CAD build for the part. Positions are in the model's coordinates, mm. A direction names the side the tool comes from. Give positions to 0.01 mm unless a question says otherwise; leave off trailing zeros. Write each loop counter-clockwise with the first axis right and the second up, starting at its lowest first coordinate (ties: lowest second). Pieces come first, ordered by that corner, then holes. Notation, with made-up numbers: (-8.75, 60.25) - (48.25, 60.25) arc R27 cw to (48.25, 76.25) - close; hole circle Ø2 at (61, 51). An arc over 180 degrees is marked (long way). Answer as a JSON object with one key per item and string values.
from build123d import *

# Parameters (mm, degrees)
BOSS_EXTRUDE1_DEPTH = 8
SKETCH10_W          = 20
SKETCH10_H          = 4.457955928
CUT_EXTRUDE1_DEPTH  = 8
SKETCH11_R          = 1.6
CUT_EXTRUDE2_DEPTH  = 17
CIRPATTERN1_START   = 27.11938858
CIRPATTERN1_DEPTH   = 8
FILLET1_R           = 4
SKETCH13_R          = 1.6
CUT_EXTRUDE3_DEPTH  = 4


# Read off the part's stored shape, not the designer's step: CirPattern1
with BuildPart() as part:
    # Sketch9 → Boss-Extrude1 (new body)
    with BuildSketch(Plane.XY.offset(35.11938858)):
        with BuildLine():
            Line((9.545521872, 41.744275524), (-57.430180647, 41.351233323))
            Line((-57.430180647, 41.351233323), (-12.111028973, 4.62462141))
            Line((-12.111028973, 4.62462141), (-5.395050947, -0.818002943))
            ThreePointArc((-5.395050947, -0.818002943), (4.336911047, 15.452862836), (9.11951655, 33.798948033))
            Line((9.11951655, 33.798948033), (11.42846507, 34.572240818))
            Line((11.42846507, 34.572240818), (11.499640251, 35.338944212))
            Line((11.499640251, 35.338944212), (9.372495407, 36.524051722))
            ThreePointArc((9.372495407, 36.524051722), (9.443412954, 37.633480095), (9.495906894, 38.743932705))
            Line((9.495906894, 38.743932705), (16.9130003, 38.787459396))
            Line((16.9130003, 38.787459396), (16.895395314, 41.78740774))
            Line((16.895395314, 41.78740774), (9.545521872, 41.744275524))
        make_face()
    extrude(amount=-BOSS_EXTRUDE1_DEPTH)

    # Sketch10 → Cut-Extrude1 (cut)
    with BuildSketch(Plane.XY.offset(35.11938858)):
        with Locations((-23.032343606, 36.517264559)):
            Rectangle(SKETCH10_W, SKETCH10_H)
    extrude(amount=-CUT_EXTRUDE1_DEPTH, mode=Mode.SUBTRACT)

    # Sketch11 → Cut-Extrude2 (cut)
    with BuildSketch(Plane(origin=(0.747199109, 41.914596091, 0), x_dir=(0.9998411421690517, -0.01782387236506677, 0), z_dir=(0.01782387236506677, 0.9998411421690517, 0))):
        with Locations(Location((-23.320690328, -31.11938858, 0), (0, 0, 180))):
            Circle(SKETCH11_R)
    extrude(amount=-CUT_EXTRUDE2_DEPTH, mode=Mode.SUBTRACT)

    # CirPattern1 outline → CirPattern1 (add)
    with BuildSketch(Plane.XY.offset(CIRPATTERN1_START)):
        with BuildLine():
            Line((-1.898240417, 0.075678285), (-1.442349939, 0.696213436))
            Line((-1.442349939, 0.696213436), (-2.655293453, 2.807609427))
            ThreePointArc((-2.655293453, 2.807609427), (-3.454215375, 1.696544027), (-4.275670815, 0.602033397))
            Line((-4.275670815, 0.602033397), (-1.898240417, 0.075678285))
        make_face()
        with BuildLine():
            ThreePointArc((9.087032741, 33.518000709), (8.913106654, 32.160616358), (8.711484025, 30.807068844))
            Line((8.711484025, 30.807068844), (11.052940174, 31.475505904))
            Line((11.052940174, 31.475505904), (11.158600181, 32.238222079))
            Line((11.158600181, 32.238222079), (9.087032741, 33.518000709))
        make_face()
        with BuildLine():
            ThreePointArc((8.666370259, 30.527871164), (8.431440362, 29.179705557), (8.169015006, 27.836621236))
            Line((8.169015006, 27.836621236), (10.538219647, 28.398843937))
            Line((10.538219647, 28.398843937), (10.678149721, 29.156022631))
            Line((10.678149721, 29.156022631), (8.666370259, 30.527871164))
        make_face()
        with BuildLine():
            ThreePointArc((8.11136298, 27.559740684), (7.81590678, 26.223534041), (7.493212091, 24.893642806))
            Line((7.493212091, 24.893642806), (9.885349689, 25.348508399))
            Line((9.885349689, 25.348508399), (10.059265414, 26.098610606))
            Line((10.059265414, 26.098610606), (8.11136298, 27.559740684))
        make_face()
        with BuildLine():
            ThreePointArc((7.423138984, 24.619642155), (7.067757013, 23.298110387), (6.685448884, 21.984115313))
            Line((6.685448884, 21.984115313), (9.095657291, 22.330699261))
            Line((9.095657291, 22.330699261), (9.303205175, 23.072200358))
            Line((9.303205175, 23.072200358), (7.423138984, 24.619642155))
        make_face()
        with BuildLine():
            ThreePointArc((6.603097126, 21.713551487), (6.188511716, 20.409380678), (5.74736721, 19.113952531))
            Line((5.74736721, 19.113952531), (8.170747547, 19.351550382))
            Line((8.170747547, 19.351550382), (8.411505736, 20.082943228))
            Line((8.411505736, 20.082943228), (6.603097126, 21.713551487))
        make_face()
        with BuildLine():
            ThreePointArc((5.652904183, 18.847375463), (5.179958002, 17.563216411), (4.680873768, 16.288988219))
            Line((4.680873768, 16.288988219), (7.112500384, 16.417117043))
            Line((7.112500384, 16.417117043), (7.385979526, 17.136915042))
            Line((7.385979526, 17.136915042), (5.652904183, 18.847375463))
        make_face()
        with BuildLine():
            ThreePointArc((4.574491474, 16.026939742), (4.04414581, 14.76540257), (3.488136265, 13.514964269))
            Line((3.488136265, 13.514964269), (5.923066749, 13.533363638))
            Line((5.923066749, 13.533363638), (6.228710981, 14.240103762))
            Line((6.228710981, 14.240103762), (4.574491474, 16.026939742))
        make_face()
        with BuildLine():
            ThreePointArc((3.370050932, 13.257977012), (2.783383741, 12.021625861), (2.171579003, 10.797519035))
            Line((2.171579003, 10.797519035), (4.604864227, 10.70615155))
            Line((4.604864227, 10.70615155), (4.942052312, 11.398397312))
            Line((4.942052312, 11.398397312), (3.370050932, 13.257977012))
        make_face()
        with BuildLine():
            ThreePointArc((2.042030645, 10.546115336), (1.400234361, 9.337463157), (0.733877956, 8.142175869))
            Line((0.733877956, 8.142175869), (3.160572137, 7.94122724))
            Line((3.160572137, 7.94122724), (3.528618722, 8.617571614))
            Line((3.528618722, 8.617571614), (2.042030645, 10.546115336))
        make_face()
        with BuildLine():
            ThreePointArc((0.593129889, 7.896866722), (-0.102491005, 6.718370166), (-0.82204467, 5.554331901))
            Line((-0.82204467, 5.554331901), (1.593126081, 5.244210567))
            Line((1.593126081, 5.244210567), (1.991283091, 5.903278845))
            Line((1.991283091, 5.903278845), (0.593129889, 7.896866722))
        make_face()
        with BuildLine():
            ThreePointArc((-0.973706371, 5.315615908), (-1.721737986, 4.169670332), (-2.493026381, 3.039247062))
            Line((-2.493026381, 3.039247062), (-0.094288024, 2.620583361))
            Line((-0.094288024, 2.620583361), (0.333170136, 3.261035952))
            Line((0.333170136, 3.261035952), (-0.973706371, 5.315615908))
        make_face()
    extrude(amount=CIRPATTERN1_DEPTH)

    # Fillet1
    fillet1_edges = [part.edges().sort_by_distance(p)[0] for p in [
        (-57.430180647, 41.351233323, 31.11938858),
    ]]
    fillet(fillet1_edges, radius=FILLET1_R)

    # Sketch13 → Cut-Extrude3 (cut)
    with BuildSketch(Plane(origin=(-0.244636188, 41.68682267, 0), x_dir=(0.9999827812112165, 0.005868328644527354, 0), z_dir=(-0.005868328644527354, 0.9999827812112165, 0))):
        with Locations(Location((12.140326638, -31.11938858, 0), (0, 0, 180))):
            Circle(SKETCH13_R)
    extrude(amount=-CUT_EXTRUDE3_DEPTH, mode=Mode.SUBTRACT)


solid = part.part
(1) Flat gauge pins, fed straight in: P1, Ø4, axis at x = -24.5, z = 30.5, coming from the +Y side; P2, Ø1.3, axis at y = 36.5, z = 31, coming from the +X side; P3, Ø4, axis at x = -23.5, z = 30.5, coming from the -Y side. Where does each tip first touch, or does it go through?
Answer key:
{"P1": "stops at y = 41.55", "P2": "stops at x = 10.58", "P3": "stops at y = 12.23"}
(2) Probe L1, parallel to Y at x = -20.5, z = 31; L2, parallel to Y at x = 11, z = 33.5; L3, parallel to Y at x = 9, z = 30.5. List the from-to ranges inside material, lowest first. Write a range as [from, to].
Answer key:
{"L1": "y = [11.42, 34.29], [38.75, 41.57]", "L2": "y = [31.46, 32.34], [34.43, 35.62], [38.75, 41.75]", "L3": "y = [22.32, 23.32], [25.18, 26.89], [28.03, 30.3], [30.89, 41.74]"}
(3) 3-axis set-ups, long thin cutter, end or side, ignore diameter. For faces 4 (the face through (-13.032, 36, 31)), 5 (the face through (6.94, 19.23, 31.06)): which of +Z, -Z, +X, -X, +Y, -Y reach the whole face in a straight line?
Answer key:
{"face 4": "+Z, -Z", "face 5": "+Z, -Z, +X"}
(4) Saw through at A-A, the plane x = -30. Give the cut face in (y, z).
Answer key:
{"outline": "(19.12, 27.12) - (34.29, 27.12) - (34.29, 35.12) - (19.12, 35.12) - close; (38.75, 27.12) - (41.51, 27.12) - (41.51, 35.12) - (38.75, 35.12) - close"}
(5) Pull direction X, two halves, no side cores. Call faces 1 (the face through (-4.838, -0.122, 31.175)), 2 (the face through (-17, 26, 35.119)), 3 (the face through (8.376, 23.835, 31.063)): pulls with the +X half, pulls with the -X half, needs draft (parallel to the pull), parting line crosses it, or undercut.
Answer key:
{"face 1": "undercut", "face 2": "needs draft", "face 3": "pulls with the +X half"}
